Can you work these out from the model? Positions are in its coordinate system, mm. A direction names the side the tool comes from. Give positions to 0.01 mm unless a question says otherwise; leave off trailing zeros. Order: outer loops, then holes, each group sorted by start corner. A loop starts at its lowest first (then second) coordinate and runs counter-clockwise, first axis right, second up. Notation, with made-up numbers: M 31,86 L 63,86 A11 cw 63,106 Z; hole C 67.25,10.25 d8. An arc over 180 degrees is marked long. Use a Markdown table: item, result. Add a question column.
from build123d import *

# Parameters (mm, degrees)
F0_W     = 5
F0_H     = 50
F0_W_2   = 15
F0_H_2   = 10
F2_DEPTH = 45


with BuildPart() as f1:
    # F0 (on Front) → F1 (revolve)
    with BuildSketch(Plane.XZ):
        with Locations((-27.5, 25)):
            Rectangle(F0_W, F0_H)
        Polygon((-25, 0), (-30, 0), (-45, 0), (-45, -10), (-30, -10), (-6.5, -10), (-6.5, -8), (-4.5, -8), (-4.5, -4), (-10, 0), align=None)
    revolve(axis=Axis((0, 0, -5), (0, 0, -1)))

    # F0 (on Front) → F2 (join, symmetric)
    with BuildSketch(Plane.XZ):
        Polygon((-25, 0), (-30, 0), (-45, 0), (-45, -10), (-30, -10), (-6.5, -10), (-6.5, -8), (-4.5, -8), (-4.5, -4), (-10, 0), align=None)
        Polygon((25, 0), (10, 0), (4.5, -4), (4.5, -8), (6.5, -8), (6.5, -10), (30, -10), (30, 0), align=None)
        with Locations((37.5, -5)):
            Rectangle(F0_W_2, F0_H_2)
    extrude(amount=F2_DEPTH, both=True)


solid = f1.part
1. If we section it at A-A, the plane x = 0: List the corners of the cut face in (y, z) for me, then the cut area to 3 significant figures.
2. On a 3-axis mill with a long thin cutter (end or side, diameter ignored), from which of +Z, -Z, +X, -X, +Y, -Y can I reach the whole of each face in a straight line? I mean faces 1 (the face through (-25, -45, -5)), 2 (the face through (5.158, -3.955, -8.986)), 3 (the face through (-23.846, 7.509, 25.35)). Say none if no direction works.
3. If we section it at C-C, the plane z = 21: List the corners of the cut face in (x, y) for me, then the cut area to 3 significant figures.
4. Will these pins go through, and if not, where does the flat tip stop? pin 1 (1.5 mm diameter, centred on x = -0.5, y = -4.5, fed in from +Z); pin 2 (15 mm diameter, centred on x = 7.5, y = 10, fed in from +Z); pin 3 (10.5 mm diameter, centred on x = 0, y = 0, fed in from -Z); pin 4 (12 mm diameter, centred on y = 24, z = 4.5, fed in from +X).
5. If we section it at D-D, the plane x = 13: List the corners of the cut face in (y, z) for me, then the cut area to 3 significant figures.
6. I need wall thicknesses on L1, parallel to Y at x = 0, z = 29.5; L2, parallel to X at y = 0, z = -6. Which ranges of each line are inside material? Lowest first, please. Write a range as [from, to].
Geometry results:
| question | item | result |
|---|---|---|
| 1 | outline | M -45,-10 L -6.5,-10 L -6.5,-8 L -4.5,-8 L -4.5,-4 L -10,0 L -25,0 L -25,50 L -30,50 L -30,0 L -45,0 Z; M 4.5,-8 L 6.5,-8 L 6.5,-10 L 45,-10 L 45,0 L 30,0 L 30,50 L 25,50 L 25,0 L 10,0 L 4.5,-4 Z |
| 1 | area | 1,280 mm^2 |
| 2 | face 1 | +Z, -Z, +X, -X, -Y |
| 2 | face 2 | -Z |
| 2 | face 3 | +Z |
| 3 | outline | C 0,0 d60; hole C 0,0 d50 |
| 3 | area | 864 mm^2 |
| 4 | pin 1 | stops at z = -3.43 |
| 4 | pin 2 | stops at z = 0 |
| 4 | pin 3 | stops at z = -8 |
| 4 | pin 4 | stops at x = 45 |
| 5 | outline | M -45,-10 L 45,-10 L 45,0 L 27.04,0 L 27.04,50 L 21.35,50 L 21.35,0 L -21.35,0 L -21.35,50 L -27.04,50 L -27.04,0 L -45,0 Z |
| 5 | area | 1,470 mm^2 |
| 6 | L1 | y = [-30, -25], [25, 30] |
| 6 | L2 | x = [-45, -4.5], [4.5, 45] |
